```python
from build123d import *

# Parameters (mm, degrees)
SKETCH1_R           = 15.25
BOSS_EXTRUDE1_DEPTH = 23.5
SKETCH2_R           = 5
BOSS_EXTRUDE2_DEPTH = 4.5
SHELL1_T            = -0.5
SKETCH3_R           = 1.75
CUT_EXTRUDE1_DEPTH  = 4.5


with BuildPart() as part:
    # Sketch1 → Boss-Extrude1 (new, symmetric)
    with BuildSketch(Plane.XY):
        Circle(SKETCH1_R)
    extrude(amount=BOSS_EXTRUDE1_DEPTH, both=True)

    # Sketch2 → Boss-Extrude2 (add)
    with BuildSketch(Plane.XY.offset(23.5)):
        Circle(SKETCH2_R)
    extrude(amount=BOSS_EXTRUDE2_DEPTH)

    # Shell1
    shell1_openings = [part.faces().sort_by_distance(p)[0] for p in [
        (0, 0, -23.5),
        (0, 0, 28),
    ]]
    offset(amount=SHELL1_T, openings=shell1_openings, kind=Kind.INTERSECTION)

    # Sketch3 → Cut-Extrude1 (cut)
    with BuildSketch(Plane.XY.offset(23.5)):
        with Locations((-10, 0)):
            Circle(SKETCH3_R)
        with Locations((0, 10)):
            Circle(SKETCH3_R)
        with Locations((10, 0)):
            Circle(SKETCH3_R)
    extrude(amount=-CUT_EXTRUDE1_DEPTH, mode=Mode.SUBTRACT)


solid = part.part
```
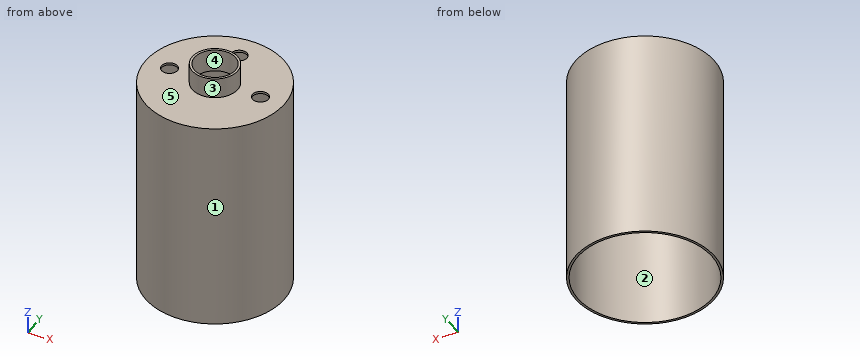
Source: CAD feature listing. Evaluate the final solid. Frame: model axes, mm. Face numbers are marked on the shaded views. A direction names the side the tool comes from. Round coordinates to 2 decimals unless told otherwise and drop trailing zeros. Loops run counter-clockwise (first coordinate to the right, second up) from the corner with the lowest first, then second, coordinate; pieces in that order, holes last.
1. Contact query for flat-ended pins moving along their axis: pin 1 (4 mm diameter, centred on x = 10, y = 0, fed in from +Z); pin 2 (4 mm diameter, centred on x = 8, z = 15.5, fed in from +Y); pin 3 (8 mm diameter, centred on x = 3, y = -9, fed in from -Z); pin 4 (6 mm diameter, centred on x = 6.5, y = -4.5, fed in from +Z). Output: stop coordinate, or through.
2. Section query B-B on y = 10. Output: boundary loops of the cut face in (x, z), and give its area (3 significant figures).
3. Ray query, L1, parallel to Y at x = 0, z = 24; L2, parallel to X at y = -0.5, z = -15.5; L3, parallel to Y at x = 0, z = -9. Return the intervals inside material, ascending.
4. Mould query, pull axis X, two halves, no side actions, for the marked faces 3, 4 and 5. Classes: released by +X, released by -X, zero draft, split by the parting line, or undercut.
5. Section query A-A on x = 0. Output: boundary loops of the cut face in (y, z).
6. Access query for the marked faces 1 and 2. Directions: +Z, -Z, +X, -X, +Y, -Y. A direction counts if a zero-diameter tool reaches every point of the face in a straight line with its end or side. Return the directions, or none.
7. Section query D-D on y = -12. Output: boundary loops of the cut face in (x, z), and give its area (3 significant figures).
Answers below:
1. pin 1: stops at z = 23.5
1. pin 2: stops at y = 14.02
1. pin 3: stops at z = 23
1. pin 4: stops at z = 28
2. outline: (-11.51, -23.5) - (-10.84, -23.5) - (-10.84, 23) - (-1.75, 23) - (-1.75, 23.5) - (-11.51, 23.5) - close; (1.75, 23) - (10.84, 23) - (10.84, -23.5) - (11.51, -23.5) - (11.51, 23.5) - (1.75, 23.5) - close
2. area: 72.2 mm2
3. L1: y = -5 to -4.5, 4.5 to 5
3. L2: x = -15.24 to -14.74, 14.74 to 15.24
3. L3: y = -15.25 to -14.75, 14.75 to 15.25
4. face 3: split by the parting line
4. face 4: undercut
4. face 5: zero draft
5. outline: (-15.25, -23.5) - (-14.75, -23.5) - (-14.75, 23) - (-4.5, 23) - (-4.5, 28) - (-5, 28) - (-5, 23.5) - (-15.25, 23.5) - close; (4.5, 23) - (8.25, 23) - (8.25, 23.5) - (5, 23.5) - (5, 28) - (4.5, 28) - close; (11.75, 23) - (14.75, 23) - (14.75, -23.5) - (15.25, -23.5) - (15.25, 23.5) - (11.75, 23.5) - close
6. face 1: +Z, -Z
6. face 2: -Z
7. outline: (-9.41, -23.5) - (-8.58, -23.5) - (-8.58, 23) - (8.58, 23) - (8.58, -23.5) - (9.41, -23.5) - (9.41, 23.5) - (-9.41, 23.5) - close
7. area: 87.0 mm2
